```python
from build123d import *

# Parameters (mm, degrees)
SKETCH1_W           = 63.5
SKETCH1_H           = 254
BOSS_EXTRUDE1_DEPTH = 3.175
SKETCH4_R           = 13.335
BOSS_EXTRUDE4_DEPTH = 3.175
SKETCH5_R           = 2
MOTOR_HOLES_DEPTH   = 227.541979167
SKETCH7_R           = 2.159
CUT_EXTRUDE2_DEPTH  = 227.541979167


with BuildPart() as part:
    # Sketch1 → Boss-Extrude1 (new body)
    with BuildSketch(Plane(origin=(0, 0, 0), x_dir=(1, 0, 0), z_dir=(0, 1, 0))):
        Polygon((-44.45, 139.7), (44.45, 139.7), (161.925, 139.7), (161.925, 120.65), (44.45, 120.65), (44.45, -120.65), (161.925, -120.65), (161.925, -139.7), (44.45, -139.7), (-44.45, -139.7), (-161.925, -139.7), (-161.925, -120.65), (-44.45, -120.65), (-44.45, 120.65), (-161.925, 120.65), (-161.925, 139.7), align=None)
        Rectangle(SKETCH1_W, SKETCH1_H, mode=Mode.SUBTRACT)
    extrude(amount=BOSS_EXTRUDE1_DEPTH)

    # Sketch4 → Boss-Extrude4 (add)
    with BuildSketch(Plane(origin=(0, 3.175, 0), x_dir=(1, 0, 0), z_dir=(0, 1, 0))):
        with Locations((161.925, 130.175)):
            Circle(SKETCH4_R)
        with Locations((-161.925, 130.175)):
            Circle(SKETCH4_R)
        with Locations((-161.925, -130.175)):
            Circle(SKETCH4_R)
        with Locations((161.925, -130.175)):
            Circle(SKETCH4_R)
    extrude(amount=-BOSS_EXTRUDE4_DEPTH)

    # Sketch5 → Motor Holes (cut, through all)
    with BuildSketch(Plane(origin=(0, 3.175, 0), x_dir=(1, 0, 0), z_dir=(0, 1, 0))):
        with Locations(Location((161.925, 130.175, 0), (0, 0, 270))):
            Circle(SKETCH5_R)
        with Locations(Location((-161.925, 130.175, 0), (0, 0, 90))):
            Circle(SKETCH5_R)
        with Locations(Location((161.925, -130.175, 0), (0, 0, 90))):
            Circle(SKETCH5_R)
        with Locations(Location((-161.925, -130.175, 0), (0, 0, 270))):
            Circle(SKETCH5_R)
        with BuildLine():
            Line((151.425, 131.425), (153.425, 131.425))
            ThreePointArc((153.425, 131.425), (154.675, 130.175), (153.425, 128.925))
            Line((153.425, 128.925), (151.425, 128.925))
            ThreePointArc((151.425, 128.925), (150.175, 130.175), (151.425, 131.425))
        make_face()
        with BuildLine():
            Line((172.425, 131.425), (170.425, 131.425))
            ThreePointArc((170.425, 131.425), (169.175, 130.175), (170.425, 128.925))
            Line((170.425, 128.925), (172.425, 128.925))
            ThreePointArc((172.425, 128.925), (173.675, 130.175), (172.425, 131.425))
        make_face()
        with BuildLine():
            Line((163.175, 139.175), (163.175, 137.175))
            ThreePointArc((163.175, 137.175), (161.925, 135.925), (160.675, 137.175))
            Line((160.675, 137.175), (160.675, 139.175))
            ThreePointArc((160.675, 139.175), (161.925, 140.425), (163.175, 139.175))
        make_face()
        with BuildLine():
            Line((163.175, 121.175), (163.175, 123.175))
            ThreePointArc((163.175, 123.175), (161.925, 124.425), (160.675, 123.175))
            Line((160.675, 123.175), (160.675, 121.175))
            ThreePointArc((160.675, 121.175), (161.925, 119.925), (163.175, 121.175))
        make_face()
        with BuildLine():
            Line((-151.425, 131.425), (-153.425, 131.425))
            ThreePointArc((-153.425, 131.425), (-154.675, 130.175), (-153.425, 128.925))
            Line((-153.425, 128.925), (-151.425, 128.925))
            ThreePointArc((-151.425, 128.925), (-150.175, 130.175), (-151.425, 131.425))
        make_face()
        with BuildLine():
            Line((-172.425, 131.425), (-170.425, 131.425))
            ThreePointArc((-170.425, 131.425), (-169.175, 130.175), (-170.425, 128.925))
            Line((-170.425, 128.925), (-172.425, 128.925))
            ThreePointArc((-172.425, 128.925), (-173.675, 130.175), (-172.425, 131.425))
        make_face()
        with BuildLine():
            Line((-163.175, 139.175), (-163.175, 137.175))
            ThreePointArc((-163.175, 137.175), (-161.925, 135.925), (-160.675, 137.175))
            Line((-160.675, 137.175), (-160.675, 139.175))
            ThreePointArc((-160.675, 139.175), (-161.925, 140.425), (-163.175, 139.175))
        make_face()
        with BuildLine():
            Line((-163.175, 121.175), (-163.175, 123.175))
            ThreePointArc((-163.175, 123.175), (-161.925, 124.425), (-160.675, 123.175))
            Line((-160.675, 123.175), (-160.675, 121.175))
            ThreePointArc((-160.675, 121.175), (-161.925, 119.925), (-163.175, 121.175))
        make_face()
        with BuildLine():
            Line((151.425, -131.425), (153.425, -131.425))
            ThreePointArc((153.425, -131.425), (154.675, -130.175), (153.425, -128.925))
            Line((153.425, -128.925), (151.425, -128.925))
            ThreePointArc((151.425, -128.925), (150.175, -130.175), (151.425, -131.425))
        make_face()
        with BuildLine():
            Line((163.175, -139.175), (163.175, -137.175))
            ThreePointArc((163.175, -137.175), (161.925, -135.925), (160.675, -137.175))
            Line((160.675, -137.175), (160.675, -139.175))
            ThreePointArc((160.675, -139.175), (161.925, -140.425), (163.175, -139.175))
        make_face()
        with BuildLine():
            Line((172.425, -131.425), (170.425, -131.425))
            ThreePointArc((170.425, -131.425), (169.175, -130.175), (170.425, -128.925))
            Line((170.425, -128.925), (172.425, -128.925))
            ThreePointArc((172.425, -128.925), (173.675, -130.175), (172.425, -131.425))
        make_face()
        with BuildLine():
            Line((163.175, -121.175), (163.175, -123.175))
            ThreePointArc((163.175, -123.175), (161.925, -124.425), (160.675, -123.175))
            Line((160.675, -123.175), (160.675, -121.175))
            ThreePointArc((160.675, -121.175), (161.925, -119.925), (163.175, -121.175))
        make_face()
        with BuildLine():
            Line((-163.175, -121.175), (-163.175, -123.175))
            ThreePointArc((-163.175, -123.175), (-161.925, -124.425), (-160.675, -123.175))
            Line((-160.675, -123.175), (-160.675, -121.175))
            ThreePointArc((-160.675, -121.175), (-161.925, -119.925), (-163.175, -121.175))
        make_face()
        with BuildLine():
            Line((-163.175, -139.175), (-163.175, -137.175))
            ThreePointArc((-163.175, -137.175), (-161.925, -135.925), (-160.675, -137.175))
            Line((-160.675, -137.175), (-160.675, -139.175))
            ThreePointArc((-160.675, -139.175), (-161.925, -140.425), (-163.175, -139.175))
        make_face()
        with BuildLine():
            Line((-172.425, -131.425), (-170.425, -131.425))
            ThreePointArc((-170.425, -131.425), (-169.175, -130.175), (-170.425, -128.925))
            Line((-170.425, -128.925), (-172.425, -128.925))
            ThreePointArc((-172.425, -128.925), (-173.675, -130.175), (-172.425, -131.425))
        make_face()
        with BuildLine():
            Line((-151.425, -131.425), (-153.425, -131.425))
            ThreePointArc((-153.425, -131.425), (-154.675, -130.175), (-153.425, -128.925))
            Line((-153.425, -128.925), (-151.425, -128.925))
            ThreePointArc((-151.425, -128.925), (-150.175, -130.175), (-151.425, -131.425))
        make_face()
    extrude(amount=-MOTOR_HOLES_DEPTH, mode=Mode.SUBTRACT)

    # Sketch7 → Cut-Extrude2 (cut, through all)
    with BuildSketch(Plane(origin=(0, 3.175, 0), x_dir=(1, 0, 0), z_dir=(0, 1, 0))):
        with Locations(Location((-38.1, 133.35, 0), (0, 0, 270))):
            Circle(SKETCH7_R)
        with Locations(Location((-38.1, 66.675, 0), (0, 0, 270))):
            Circle(SKETCH7_R)
        with Locations(Location((-38.1, 0, 0), (0, 0, 270))):
            Circle(SKETCH7_R)
        with Locations(Location((-38.1, -66.675, 0), (0, 0, 270))):
            Circle(SKETCH7_R)
        with Locations(Location((-38.1, -133.35, 0), (0, 0, 270))):
            Circle(SKETCH7_R)
        with Locations(Location((38.1, -133.35, 0), (0, 0, 90))):
            Circle(SKETCH7_R)
        with Locations(Location((38.1, -66.675, 0), (0, 0, 90))):
            Circle(SKETCH7_R)
        with Locations(Location((38.1, 0, 0), (0, 0, 90))):
            Circle(SKETCH7_R)
        with Locations(Location((38.1, 66.675, 0), (0, 0, 90))):
            Circle(SKETCH7_R)
        with Locations(Location((38.1, 133.35, 0), (0, 0, 90))):
            Circle(SKETCH7_R)
        with Locations(Location((0, 133.35, 0), (0, 0, 270))):
            Circle(SKETCH7_R)
        with Locations(Location((0, -133.35, 0), (0, 0, 90))):
            Circle(SKETCH7_R)
    extrude(amount=-CUT_EXTRUDE2_DEPTH, mode=Mode.SUBTRACT)


solid = part.part
```
Work out the finished part from the listing and answer in its coordinate system (mm). Give positions to 0.01 mm unless a question says otherwise; leave off trailing zeros. Write each loop counter-clockwise with the first axis right and the second up, starting at its lowest first coordinate (ties: lowest second). Pieces come first, ordered by that corner, then holes. Notation, with made-up numbers: (64.25, 77.25) - (107.25, 77.25) arc R33 cw to (107.25, 113.25) - close; hole circle Ø5 at (-6, 59). An arc over 180 degrees is marked (long way). Use one line per item in the form item = value.
1. A cutting plane is placed at A-A (x = 14.5). Write down the section's boundary in (y, z) (3 decimals), and give its area (3 significant figures).
Filled in:
outline = (0, -139.7) - (3.175, -139.7) - (3.175, -127) - (0, -127) - close; (0, 127) - (3.175, 127) - (3.175, 139.7) - (0, 139.7) - close
area = 80.6 mm^2
2. Determine the mould class of faces 1 (the face through (-40, 3.175, 10)), 2 (the face through (-175.253, 1.61, 129.737)), 3 (the face through (-175.253, 1.61, -130.613)) for opening direction Z: released by +Z, released by -Z, zero draft, split by the parting line, or undercut.
Filled in:
face_1 = zero draft
face_2 = undercut
face_3 = undercut
3. A cutting plane is placed at C-C (y = 2.6). State how many separate pieces and enclosed holes the cut face has, and give its area (3 significant figures).
Filled in:
separate_pieces = 1
enclosed_holes = 33
area = 18,600 mm^2
4. Consider L1, parallel to Z at x = 152, y = 1.8 (3 decimals); L2, parallel to Z at x = 38.1, y = 2.3; L3, parallel to X at y = 2.5, z = 52. Determine where each line is inside the solid, lowest interval first.
Filled in:
L1 = -139.7 to -131.425, -128.925 to -120.65, 120.65 to 128.925, 131.425 to 139.7
L2 = -139.7 to -135.51, -131.19 to -68.83, -64.52 to -2.16, 2.16 to 64.52, 68.83 to 131.19, 135.51 to 139.7
L3 = -44.45 to -31.75, 31.75 to 44.45
5. A cutting plane is placed at B-B (z = 86). Write down the section's boundary in (x, y) (3 decimals).
Filled in:
outline = (-44.45, 0) - (-31.75, 0) - (-31.75, 3.175) - (-44.45, 3.175) - close; (31.75, 0) - (44.45, 0) - (44.45, 3.175) - (31.75, 3.175) - close
6. Each of these flat-tipped pins is pushed along its axis until it touches: pin 1 Ø1.6 at (x, y) = (152.5, 1.5) entering from +Z; pin 2 Ø1.6 at (x, y) = (152.5, 2) entering from -Z; pin 3 Ø4 at (x, z) = (-38.1, 66.675) entering from +Y; pin 4 Ø1.5 at (y, z) = (0.5, -106.5) entering from -X. Where does it stop, or does it pass through?
Filled in:
pin_1 = 140.35
pin_2 = -140.35
pin_3 = through
pin_4 = -44.45
